Source: CAD feature listing. Evaluate the final solid. Frame: model axes, mm. Face numbers are marked on the shaded views. A direction names the side the tool comes from. Round coordinates to 2 decimals unless told otherwise and drop trailing zeros. Order: outer loops, then holes, each group sorted by start corner. A loop starts at its lowest first (then second) coordinate and runs counter-clockwise, first axis right, second up. Notation, with made-up numbers: M 56.5,78 L 87.5,78 A31 ccw 87.5,112 Z; hole C 38,-27.75 d5. An arc over 180 degrees is marked long. Use one line per item in the form item = value. Start each with the question number.
Q1. Contact query for flat-ended pins moving along their axis: pin 1 (4 mm diameter, centred on x = -20.27, z = 4.5, fed in from +Y); pin 2 (5 mm diameter, centred on y = -2, z = 7.5, fed in from +X); pin 3 (3 mm diameter, centred on y = 5, z = 14.5, fed in from +X); pin 4 (9.5 mm diameter, centred on x = -11, z = 12.5, fed in from +Y). Output: stop coordinate, or through.
Q2. Section A-A (z = 5.75). Return the cut outline in (x, y).
Q3. Material intervals for probe 1 along X at (y, z) = (0, 14.5); probe 2 along X at (y, z) = (2.5, 2.5); probe 3 along X at (y, z) = (-2, 14.5), sorted ascending.
Q4. Section D-D (x = -13). Return the cut outline in (y, z).
Q5. Pull-direction query (X, two-part tool) for the marked faces 3, 4 and 5; classes: pulls with the +X half, pulls with the -X half, needs draft (parallel to the pull), parting line crosses it, or undercut.
Q6. Reachability of the marked faces 1 and 2 from +Z, -Z, +X, -X, +Y, -Y: full face, straight path, thin tool, end or side. Return the list, or none.
Q7. Section B-B (y = 4). Return the cut outline in (x, z), plus the area to 3 significant figures.
Q8. Section C-C (z = 14.5). Return the cut outline in (x, y).
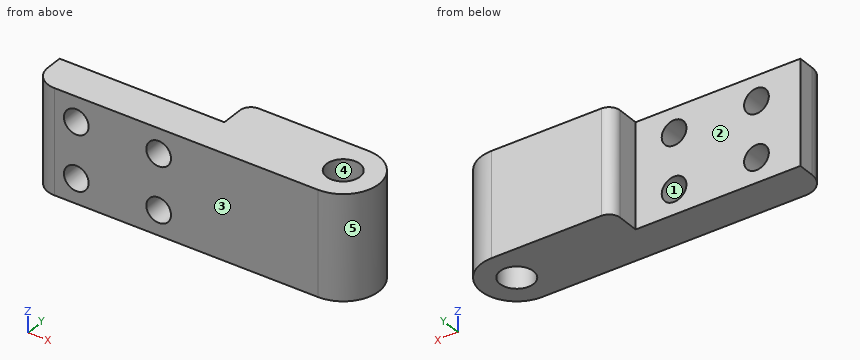
from build123d import *

# Parameters (mm, degrees)
SKETCH_1_R          = 3.05
EXTRUDE_1_DEPTH     = 19
SKETCH_2_R          = 2.25
CUT_EXTRUDE_1_DEPTH = 20
FILLET_1_R          = 4
FILLET_2_R          = 2


with BuildPart() as part:
    # 草图1 → 凸台-拉伸1 (new body)
    with BuildSketch(Plane.XY):
        with BuildLine():
            Line((1.728973827, 8.951048951), (23.728973827, 8.951048951))
            ThreePointArc((23.728973827, 8.951048951), (30.228973827, 2.451048951), (23.728973827, -4.048951049))
            Line((23.728973827, -4.048951049), (-28.271026173, -4.048951049))
            Line((-28.271026173, -4.048951049), (-28.271026173, 2.951048951))
            Line((-28.271026173, 2.951048951), (1.728973827, 2.951048951))
            Line((1.728973827, 2.951048951), (1.728973827, 8.951048951))
        make_face()
        with Locations((23.728973827, 2.451048951)):
            Circle(SKETCH_1_R, mode=Mode.SUBTRACT)
    extrude(amount=EXTRUDE_1_DEPTH)

    # 草图2 → 切除-拉伸1 (cut)
    with BuildSketch(Plane(origin=(0, 2.951048951, 0), x_dir=(1, 0, 0), z_dir=(0, 1, 0))):
        with Locations((-20.271026173, -4.5)):
            Circle(SKETCH_2_R)
        with Locations((-5.271026173, -4.5)):
            Circle(SKETCH_2_R)
        with Locations((-5.271026173, -14.5)):
            Circle(SKETCH_2_R)
        with Locations((-20.271026173, -14.5)):
            Circle(SKETCH_2_R)
    extrude(amount=-CUT_EXTRUDE_1_DEPTH, mode=Mode.SUBTRACT)

    # 圆角1
    fillet_1_edges = [part.edges().sort_by_distance(p)[0] for p in [
        (-28.271026173, -4.048951049, 9.5),
    ]]
    fillet(fillet_1_edges, radius=FILLET_1_R)

    # 圆角2
    fillet_2_edges = [part.edges().sort_by_distance(p)[0] for p in [
        (1.728973827, 8.951048951, 9.5),
    ]]
    fillet(fillet_2_edges, radius=FILLET_2_R)


solid = part.part
Results list:
q1.pin_1 = through
q1.pin_2 = 29.93
q1.pin_3 = 30.14
q1.pin_4 = 2.95
q2.outline = M -28.27,-0.05 A4 ccw -24.27,-4.05 L -22.14,-4.05 L -22.14,2.95 L -28.27,2.95 Z; M -18.4,-4.05 L -7.14,-4.05 L -7.14,2.95 L -18.4,2.95 Z; M -3.4,-4.05 L 23.73,-4.05 A6.5 ccw 23.73,8.95 L 3.73,8.95 A2 ccw 1.73,6.95 L 1.73,2.95 L -3.4,2.95 Z; hole C 23.73,2.45 d6.1
q3.probe_1 = -28.27 to -22.52, -18.02 to -7.52, -3.02 to 21.91, 25.54 to 29.75
q3.probe_2 = -28.27 to -21.3, -19.24 to -6.3, -4.24 to 20.68, 26.78 to 30.23
q3.probe_3 = -27.76 to -22.52, -18.02 to -7.52, -3.02 to 28.47
q4.outline = M -4.05,0 L 2.95,0 L 2.95,19 L -4.05,19 Z
q5.face_3 = needs draft
q5.face_4 = undercut
q5.face_5 = pulls with the +X half
q6.face_1 = +Y, -Y
q6.face_2 = +Z, -Z, -X, +Y
q7.outline = M 1.73,0 L 21.1,0 L 21.1,19 L 1.73,19 Z; M 26.36,0 L 30.04,0 L 30.04,19 L 26.36,19 Z
q7.area = 438 mm2
q8.outline = M -28.27,-0.05 A4 ccw -24.27,-4.05 L -22.52,-4.05 L -22.52,2.95 L -28.27,2.95 Z; M -18.02,-4.05 L -7.52,-4.05 L -7.52,2.95 L -18.02,2.95 Z; M -3.02,-4.05 L 23.73,-4.05 A6.5 ccw 23.73,8.95 L 3.73,8.95 A2 ccw 1.73,6.95 L 1.73,2.95 L -3.02,2.95 Z; hole C 23.73,2.45 d6.1
